For this review, use the dimensioned drawing (mm, ordinates from the lowest corner) and the shaded views. Give positions to 0.01 mm unless a question says otherwise; leave off trailing zeros. Order: outer loops, then holes, each group sorted by start corner. A loop starts at its lowest first (then second) coordinate and runs counter-clockwise, first axis right, second up. Notation, with made-up numbers: (11.5, 80.25) - (69.5, 80.25) arc R20 ccw to (69.5, 107.25) - close; hole circle Ø10 at (58.5, 42.5). An arc over 180 degrees is marked (long way). One line per item, written item: value.
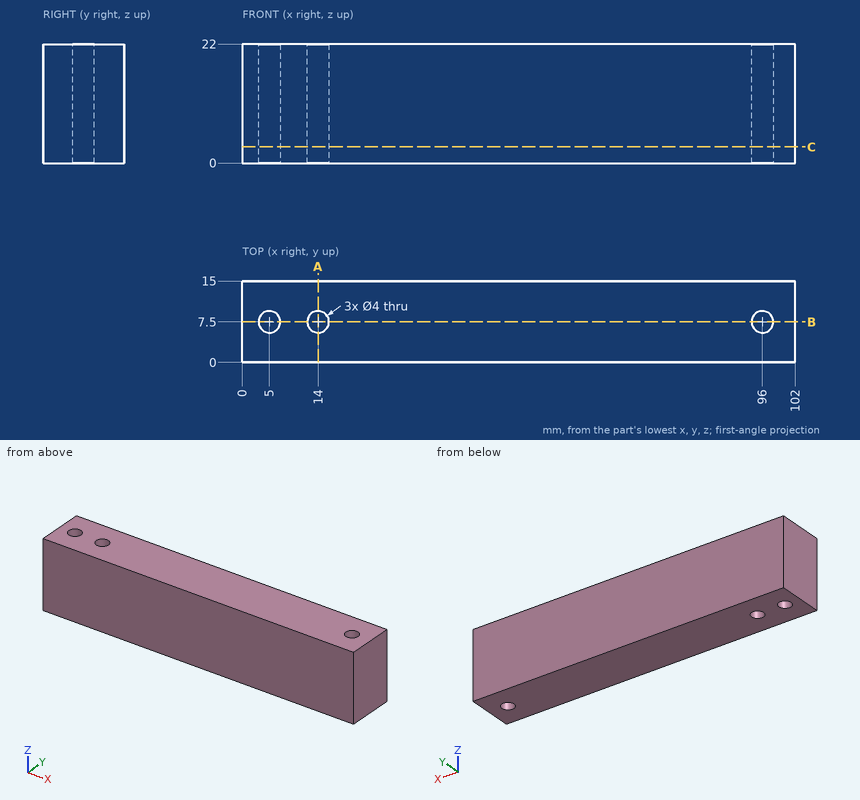
(1) Take a section at C-C (z = 3). Write out the cut boundary in (x, y).
Answers below:
outline: (0, 0) - (102, 0) - (102, 15) - (0, 15) - close; hole circle Ø4 at (5, 7.5); hole circle Ø4 at (14, 7.5); hole circle Ø4 at (96, 7.5)
(2) Wall thickness on line 1 (Y direction, x = 14, z = 14.5); line 2 (X direction, y = 5.75, z = 13); line 3 (X direction, y = 9, z = 12): over which ranges is each line inside the solid? List them lowest first. Write a range as from..to.
Answers below:
line 1: y = 0..5.5, 9.5..15
line 2: x = 0..4.03, 5.97..13.03, 14.97..95.03, 96.97..102
line 3: x = 0..3.68, 6.32..12.68, 15.32..94.68, 97.32..102
(3) Take a section at A-A (x = 14). Write out the cut boundary in (y, z), then the cut area to 3 significant figures.
Answers below:
outline: (0, 0) - (5.5, 0) - (5.5, 22) - (0, 22) - close; (9.5, 0) - (15, 0) - (15, 22) - (9.5, 22) - close
area: 242 mm^2
(4) Take a section at B-B (y = 7.5). Write out the cut boundary in (x, z).
Answers below:
outline: (0, 0) - (3, 0) - (3, 22) - (0, 22) - close; (7, 0) - (12, 0) - (12, 22) - (7, 22) - close; (16, 0) - (94, 0) - (94, 22) - (16, 22) - close; (98, 0) - (102, 0) - (102, 22) - (98, 22) - close
